Work out the finished part from the listing and answer in its coordinate system (mm). Give positions to 0.01 mm unless a question says otherwise; leave off trailing zeros. Loops run counter-clockwise (first coordinate to the right, second up) from the corner with the lowest first, then second, coordinate; pieces in that order, holes last.
from build123d import *

# Parameters (mm, degrees)
SKETCH1_W           = 5.4
SKETCH1_H           = 3.6
BOSS_EXTRUDE1_DEPTH = 5


with BuildPart() as part:
    # Sketch1 → Boss-Extrude1 (new body)
    with BuildSketch(Plane(origin=(0, 0, 0), x_dir=(1, 0, 0), z_dir=(0, 1, 0))):
        with BuildLine():
            ThreePointArc((34.042513552, 0), (26.590386774, 22.649879577), (7.14560225, 36.450299612))
            Line((7.14560225, 36.450299612), (7.14560225, 31.202638223))
            ThreePointArc((7.14560225, 31.202638223), (6.852709032, 30.495531442), (6.14560225, 30.202638223))
            Line((6.14560225, 30.202638223), (-14.35439775, 30.202638223))
            ThreePointArc((-14.35439775, 30.202638223), (-15.061504531, 30.495531442), (-15.35439775, 31.202638223))
            Line((-15.35439775, 31.202638223), (-15.35439775, 36.450299612))
            ThreePointArc((-15.35439775, 36.450299612), (-26.754277326, -30.694784524), (34.042513552, 0))
        make_face()
        with Locations((-4.10439775, 0)):
            Rectangle(SKETCH1_W, SKETCH1_H, mode=Mode.SUBTRACT)
    extrude(amount=BOSS_EXTRUDE1_DEPTH)


solid = part.part
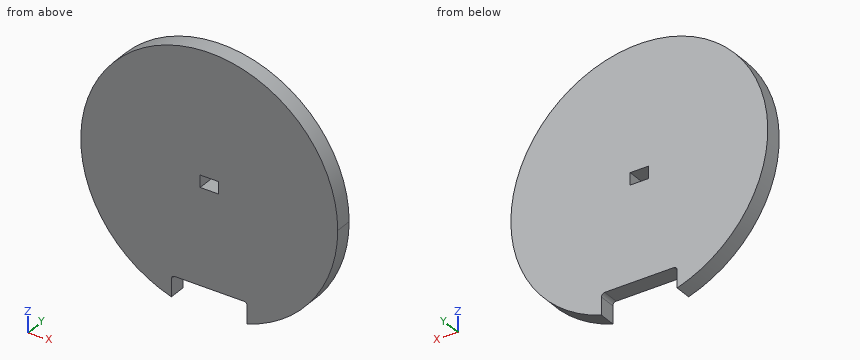
Item 1: Find section A-A, the plane y = 2.4. Write down the section's boundary in (x, z), plus the area to 3 significant figures.
Item 2: Find section B-B, the plane z = 20. Write down the section's boundary in (x, y), plus the area to 3 significant figures.
Item 3: Consider line 1 (Z direction, x = -1.5, y = 1.05); line 2 (X direction, y = 2.95, z = 32); line 3 (X direction, y = 3.8, z = -31). Determine where each line is inside the solid, lowest interval first.
Item 4: Flat-ended cylindrical pins translate along their axes: pin 1 Ø4 at (x, z) = (-10.5, -15.5) entering from -Y; pin 2 Ø1 at (x, y) = (-30, 4) entering from +Z; pin 3 Ø1.5 at (x, y) = (-29, 3) entering from -Z; pin 4 Ø1.8 at (y, z) = (2, -0.5) entering from -X. Find the tip coordinate at first contact, or state that the pin passes through.
Item 5: Find section C-C, the plane x = 21. Write down the section's boundary in (y, z).
Ans:
1. outline: (-15.35, -36.45) - (-15.35, -31.2) arc R1 cw to (-14.35, -30.2) - (6.15, -30.2) arc R1 cw to (7.15, -31.2) - (7.15, -36.45) arc R38.15 ccw (long way) to start; hole (-6.8, -1.8) - (-1.4, -1.8) - (-1.4, 1.8) - (-6.8, 1.8) - close
1. area: 4,390 mm2
2. outline: (-36.59, 0) - (28.38, 0) - (28.38, 5) - (-36.59, 5) - close
2. area: 325 mm2
3. line 1: z = -30.2 to -1.8, 1.8 to 38.06
3. line 2: x = -24.87 to 16.66
3. line 3: x = -26.33 to -15.33, 7.12 to 18.13
4. pin 1: stops at y = 0
4. pin 2: stops at z = 28.46
4. pin 3: stops at z = -29.53
4. pin 4: stops at x = -42.25
5. outline: (0, -28.72) - (5, -28.72) - (5, 28.72) - (0, 28.72) - close
